Could you check a few things on this model? Use its own coordinates, in mm. Face numbers are marked on the shaded views. Coordinates: 2 decimals unless noted, no trailing zeros. Order: outer loops, then holes, each group sorted by start corner. A loop starts at its lowest first (then second) coordinate and runs counter-clockwise, first axis right, second up. Notation, with made-up numbers: (17, 70) -> (23, 70) arc R34 cw to (23, 108) -> close; hole circle Ø2 at (-7, 8.5). An arc over 180 degrees is marked (long way). Put each result on its own line as item: value. Start each with the question number.
Q1. If we section it at A-A (x = 3): Please give me the cut outline in (y, z).
Q2. Please list where these lines run through material, in increasing order: line 1 along Y through (x, z) = (19.5, 27); line 2 along Y through (x, z) = (24.75, 18.5); line 3 along Z through (x, y) = (12.25, 33).
Q3. If we section it at C-C (y = 37): Please give me the cut outline in (x, z), and give its area (3 significant figures).
Q4. Will these pins go through, and if not, where does the flat tip stop? pin 1 (10 mm diameter, centred on y = 27, z = 16, fed in from -X); pin 2 (1 mm diameter, centred on x = 19, y = 32.5, fed in from +Z).
Q5. If we section it at B-B (z = 22): Please give me the cut outline in (x, y).
Q6. If we section it at D-D (z = 14): Please give me the cut outline in (x, y).
Q7. We'd pull the mould along Y, two halves only. Please class the marked faces 1, 2, 3 and 4: +Y half, -Y half, draft (parallel to the pull), parting line (faces both ways), or undercut.
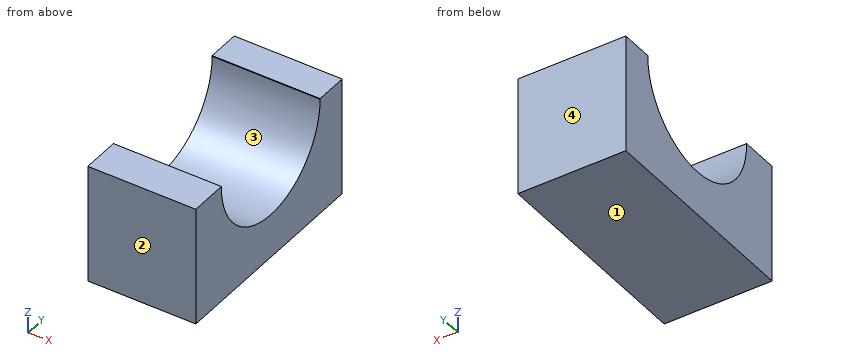
from build123d import *

# Parameters (mm, degrees)
F0_W     = 51.479302
F0_H     = 27.910465
F1_DEPTH = 25.4
F3_DEPTH = 25.4


with BuildPart() as f1:
    # F0 (on Right) → F1 (new body)
    with BuildSketch(Plane.YZ):
        with Locations((25.739651, 13.955232)):
            Rectangle(F0_W, F0_H)
    extrude(amount=F1_DEPTH)

    # F2 (on face) → F3 (cut)
    with BuildSketch(Plane.YZ.offset(25.4)):
        with BuildLine():
            ThreePointArc((8.993372, 27.910465), (26.271278, 10.366066), (43.7273, 27.733256))
            ThreePointArc((43.7273, 27.733256), (43.727074, 27.821862), (43.726396, 27.910465))
            Line((43.726396, 27.910465), (8.993372, 27.910465))
        make_face()
        with BuildLine():
            Line((8.993372, 27.910465), (43.726396, 27.910465))
            ThreePointArc((43.726396, 27.910465), (26.359884, 45.100672), (8.993372, 27.910465))
        make_face()
    extrude(amount=-F3_DEPTH, mode=Mode.SUBTRACT)


solid = f1.part
The answers:
1. outline: (0, 0) -> (51.48, 0) -> (51.48, 27.91) -> (43.73, 27.91) arc R17.37 cw to (43.73, 27.73) arc R17.37 cw (long way) to (8.99, 27.91) -> (0, 27.91) -> close
2. line 1: 0 to 9.01, 43.71 to 51.48
2. line 2: 0 to 11.65, 41.07 to 51.48
2. line 3: 0 to 11.69
3. outline: (0, 0) -> (25.4, 0) -> (25.4, 14.01) -> (0, 14.01) -> close
3. area: 356 mm^2
4. pin 1: through
4. pin 2: z = 11.69
5. outline: (0, 0) -> (25.4, 0) -> (25.4, 9.97) -> (0, 9.97) -> close; (0, 42.75) -> (25.4, 42.75) -> (25.4, 51.48) -> (0, 51.48) -> close
6. outline: (0, 0) -> (25.4, 0) -> (25.4, 15.73) -> (0, 15.73) -> close; (0, 36.99) -> (25.4, 36.99) -> (25.4, 51.48) -> (0, 51.48) -> close
7. face 1: draft
7. face 2: -Y half
7. face 3: undercut
7. face 4: +Y half
